from build123d import *

# Parameters (mm, degrees)
BOSS_EXTRUDE1_DEPTH     = 12.5
SKETCH3_R               = 20
BOSS_EXTRUDE2_DEPTH     = 20
CUT_EXTRUDE1_DEPTH      = 65.745656225
CUT_EXTRUDE1_DEPTH_BACK = 65.745656225


with BuildPart() as part:
    # Sketch2 → Boss-Extrude1 (new, symmetric)
    with BuildSketch(Plane.XY):
        with BuildLine():
            Line((1.5, 36), (-1.5, 36))
            ThreePointArc((-1.5, 36), (-3.242504384, 33.062509074), (-4, 29.732137495))
            ThreePointArc((-4, 29.732137495), (-5.85270966, 29.423558412), (-7.682478298, 28.999647019))
            ThreePointArc((-7.682478298, 28.999647019), (-9.656791021, 31.786628134), (-12.390784266, 33.833688319))
            Line((-12.390784266, 33.833688319), (-15.162422864, 32.685638022))
            ThreePointArc((-15.162422864, 32.685638022), (-15.64815789, 29.30492272), (-15.073514558, 25.93817956))
            ThreePointArc((-15.073514558, 25.93817956), (-16.667106991, 24.944088369), (-18.195368917, 23.852223166))
            ThreePointArc((-18.195368917, 23.852223166), (-21.085927531, 25.671521208), (-24.395183951, 26.516504294))
            Line((-24.395183951, 26.516504294), (-26.516504294, 24.395183951))
            ThreePointArc((-26.516504294, 24.395183951), (-25.671521208, 21.085927531), (-23.852223166, 18.195368917))
            ThreePointArc((-23.852223166, 18.195368917), (-24.944088369, 16.667106991), (-25.93817956, 15.073514558))
            ThreePointArc((-25.93817956, 15.073514558), (-29.30492272, 15.64815789), (-32.685638022, 15.162422864))
            Line((-32.685638022, 15.162422864), (-33.833688319, 12.390784266))
            ThreePointArc((-33.833688319, 12.390784266), (-31.786628134, 9.656791021), (-28.999647019, 7.682478298))
            ThreePointArc((-28.999647019, 7.682478298), (-29.423558412, 5.85270966), (-29.732137495, 4))
            ThreePointArc((-29.732137495, 4), (-33.062509074, 3.242504384), (-36, 1.5))
            Line((-36, 1.5), (-36, -1.5))
            ThreePointArc((-36, -1.5), (-33.062509074, -3.242504384), (-29.732137495, -4))
            ThreePointArc((-29.732137495, -4), (-29.423558412, -5.85270966), (-28.999647019, -7.682478298))
            ThreePointArc((-28.999647019, -7.682478298), (-31.786628134, -9.656791021), (-33.833688319, -12.390784266))
            Line((-33.833688319, -12.390784266), (-32.685638022, -15.162422864))
            ThreePointArc((-32.685638022, -15.162422864), (-29.30492272, -15.64815789), (-25.93817956, -15.073514558))
            ThreePointArc((-25.93817956, -15.073514558), (-21.213203436, -21.213203436), (-15.073514558, -25.93817956))
            ThreePointArc((-15.073514558, -25.93817956), (-15.64815789, -29.30492272), (-15.162422864, -32.685638022))
            Line((-15.162422864, -32.685638022), (-12.390784266, -33.833688319))
            ThreePointArc((-12.390784266, -33.833688319), (-9.656791021, -31.786628134), (-7.682478298, -28.999647019))
            ThreePointArc((-7.682478298, -28.999647019), (-5.85270966, -29.423558412), (-4, -29.732137495))
            ThreePointArc((-4, -29.732137495), (-3.242504384, -33.062509074), (-1.5, -36))
            Line((-1.5, -36), (1.5, -36))
            ThreePointArc((1.5, -36), (3.242504384, -33.062509074), (4, -29.732137495))
            ThreePointArc((4, -29.732137495), (5.85270966, -29.423558412), (7.682478298, -28.999647019))
            ThreePointArc((7.682478298, -28.999647019), (9.656791021, -31.786628134), (12.390784266, -33.833688319))
            Line((12.390784266, -33.833688319), (15.162422864, -32.685638022))
            ThreePointArc((15.162422864, -32.685638022), (15.64815789, -29.30492272), (15.073514558, -25.93817956))
            ThreePointArc((15.073514558, -25.93817956), (16.667106991, -24.944088369), (18.195368917, -23.852223166))
            ThreePointArc((18.195368917, -23.852223166), (21.085927531, -25.671521208), (24.395183951, -26.516504294))
            Line((24.395183951, -26.516504294), (26.516504294, -24.395183951))
            ThreePointArc((26.516504294, -24.395183951), (25.671521208, -21.085927531), (23.852223166, -18.195368917))
            ThreePointArc((23.852223166, -18.195368917), (24.944088369, -16.667106991), (25.93817956, -15.073514558))
            ThreePointArc((25.93817956, -15.073514558), (29.30492272, -15.64815789), (32.685638022, -15.162422864))
            Line((32.685638022, -15.162422864), (33.833688319, -12.390784266))
            ThreePointArc((33.833688319, -12.390784266), (31.786628134, -9.656791021), (28.999647019, -7.682478298))
            ThreePointArc((28.999647019, -7.682478298), (29.423558412, -5.85270966), (29.732137495, -4))
            ThreePointArc((29.732137495, -4), (33.062509074, -3.242504384), (36, -1.5))
            Line((36, -1.5), (36, 1.5))
            ThreePointArc((36, 1.5), (33.062509074, 3.242504384), (29.732137495, 4))
            ThreePointArc((29.732137495, 4), (29.423558412, 5.85270966), (28.999647019, 7.682478298))
            ThreePointArc((28.999647019, 7.682478298), (31.786628134, 9.656791021), (33.833688319, 12.390784266))
            Line((33.833688319, 12.390784266), (32.685638022, 15.162422864))
            ThreePointArc((32.685638022, 15.162422864), (29.30492272, 15.64815789), (25.93817956, 15.073514558))
            ThreePointArc((25.93817956, 15.073514558), (24.944088369, 16.667106991), (23.852223166, 18.195368917))
            ThreePointArc((23.852223166, 18.195368917), (25.671521208, 21.085927531), (26.516504294, 24.395183951))
            Line((26.516504294, 24.395183951), (24.395183951, 26.516504294))
            ThreePointArc((24.395183951, 26.516504294), (21.085927531, 25.671521208), (18.195368917, 23.852223166))
            ThreePointArc((18.195368917, 23.852223166), (16.667106991, 24.944088369), (15.073514558, 25.93817956))
            ThreePointArc((15.073514558, 25.93817956), (15.64815789, 29.30492272), (15.162422864, 32.685638022))
            Line((15.162422864, 32.685638022), (12.390784266, 33.833688319))
            ThreePointArc((12.390784266, 33.833688319), (9.656791021, 31.786628134), (7.682478298, 28.999647019))
            ThreePointArc((7.682478298, 28.999647019), (5.85270966, 29.423558412), (4, 29.732137495))
            ThreePointArc((4, 29.732137495), (3.242504384, 33.062509074), (1.5, 36))
        make_face()
    extrude(amount=BOSS_EXTRUDE1_DEPTH, both=True)

    # Sketch3 → Boss-Extrude2 (add, symmetric)
    with BuildSketch(Plane.XY):
        Circle(SKETCH3_R)
    extrude(amount=BOSS_EXTRUDE2_DEPTH, both=True)

    # Sketch4 → Cut-Extrude1 (cut, two sides: drawn at the far end of the back side and taken through both)
    with BuildSketch(Plane.XY.offset(20).offset(-CUT_EXTRUDE1_DEPTH_BACK)):
        with BuildLine():
            Line((4, 15), (4, 10.683441748))
            ThreePointArc((4, 10.683441748), (0, -11.407713513), (-4, 10.683441748))
            Line((-4, 10.683441748), (-4, 15))
            Line((-4, 15), (4, 15))
        make_face()
    extrude(amount=CUT_EXTRUDE1_DEPTH + CUT_EXTRUDE1_DEPTH_BACK, mode=Mode.SUBTRACT)


solid = part.part
Can you work these out from the model? Positions are in its coordinate system, mm. A direction names the side the tool comes from. Round coordinates to 2 decimals unless told otherwise and drop trailing zeros. Loops run counter-clockwise (first coordinate to the right, second up) from the corner with the lowest first, then second, coordinate; pieces in that order, holes last. Notation, with made-up numbers: (41, -6.5) - (67, -6.5) arc R16 cw to (67, 19.5) - close; hole circle Ø1 at (-12, -32.5). An arc over 180 degrees is marked (long way). Use CSV: the item, a comma, the result in double quotes. Start each with the question number.
1) Please list where these lines run through material, in increasing order: probe 1 along X at (y, z) = (0, -4); probe 2 along Y at (x, z) = (-0.5, -16); probe 3 along Z at (x, y) = (-26, -12). Write a range as [from, to].
2) We'd pull the mould along X, two halves only. Please class faces 6 (the flat face through (0, -36, 0)), 7 (the cylindrical face through (29.43, 5.83, 0.18)), 8 (the cylindrical face through (5.88, 29.42, 0.18)), 9 (the cylindrical face through (-25.69, 21.13, 0.18)): released by +X, released by -X, zero draft, split by the parting line, or undercut.
3) If we section it at C-C on z = -14: Write out the boundary of the cut face in (x, y), plus the area to 3 significant figures.
4) If we section it at B-B on x = 0: Write out the boundary of the cut face in (y, z).
5) For pin 1 Ø6 at (y, z) = (23, -12) entering from +X; pin 2 Ø5 at (x, z) = (-24.5, 0) entering from +Y; pin 3 Ø6 at (x, z) = (9.5, 5) entering from -Y, each with a flat end and sliding along its axis, tell me the tip position at first contact or that it passes through.
6) If we section it at A-A on y = 0: Write out the boundary of the cut face in (x, z), plus the area to 3 significant figures.
7) For faces 1 (the cylindrical face through (24.959, 16.645, 0.175)), 2 (the cylindrical face through (-9.62, 31.75, 0.18)), 3 (the cylindrical face through (5.83, -29.43, 0.18)), 4 (the cylindrical face through (31.82, -9.69, 0.18)), 5 (the cylindrical face through (-31.82, 9.69, 0.18)), which set-ups out of +Z, -Z, +X, -X, +Y, -Y let a thin tool reach every point of the face, with its end or its side?
Geometry results:
1,probe 1,"x = [-36, -11.41], [11.41, 36]"
1,probe 2,"y = [-19.99, -11.4], [15, 19.99]"
1,probe 3,"z = [-12.5, 12.5]"
2,face 6,"zero draft"
2,face 7,"released by +X"
2,face 8,"undercut"
2,face 9,"released by -X"
3,outline,"circle Ø40 at (0, 0); hole (-4, 10.68) arc R11.41 ccw (long way) to (4, 10.68) - (4, 15) - (-4, 15) - close"
3,area,"817 mm2"
4,outline,"(-36, -12.5) - (-20, -12.5) - (-20, -20) - (-11.41, -20) - (-11.41, 20) - (-20, 20) - (-20, 12.5) - (-36, 12.5) - close; (15, -20) - (20, -20) - (20, -12.5) - (36, -12.5) - (36, 12.5) - (20, 12.5) - (20, 20) - (15, 20) - close"
5,pin 1,"stops at x = 26.52"
5,pin 2,"stops at y = 26.52"
5,pin 3,"stops at y = -33.83"
6,outline,"(-36, -12.5) - (-20, -12.5) - (-20, -20) - (-11.41, -20) - (-11.41, 20) - (-20, 20) - (-20, 12.5) - (-36, 12.5) - close; (11.41, -20) - (20, -20) - (20, -12.5) - (36, -12.5) - (36, 12.5) - (20, 12.5) - (20, 20) - (11.41, 20) - close"
6,area,"1,490 mm2"
7,face 1,"+Z, -Z"
7,face 2,"+Z, -Z, +Y"
7,face 3,"+Z, -Z, -Y"
7,face 4,"+Z, -Z, +X"
7,face 5,"+Z, -Z, -X"
